from build123d import *

# Parameters (mm, degrees)
SKETCH1_R           = 11.1125
BOSS_EXTRUDE1_DEPTH = 38.1
SKETCH2_R           = 6.35
CUT_EXTRUDE1_DEPTH  = 25.4
SKETCH3_W           = 3.175
SKETCH3_H           = 1.5875
CUT_EXTRUDE2_DEPTH  = 25.4
CHAMFER2_SIZE       = 0.635
CHAMFER3_SIZE       = 1.27


with BuildPart() as part:
    # Sketch1 → Boss-Extrude1 (new body)
    with BuildSketch(Plane(origin=(0, 0, 0), x_dir=(0, 0, -1), z_dir=(1, 0, 0))):
        with Locations(Location((0, 0, 0), (0, 0, 180))):
            Circle(SKETCH1_R)
    extrude(amount=BOSS_EXTRUDE1_DEPTH)

    # Sketch2 → Cut-Extrude1 (cut)
    with BuildSketch(Plane(origin=(38.1, 0, 0), x_dir=(0, 0, -1), z_dir=(1, 0, 0))):
        Circle(SKETCH2_R)
    extrude(amount=-CUT_EXTRUDE1_DEPTH, mode=Mode.SUBTRACT)

    # Sketch3 → Cut-Extrude2 (cut)
    with BuildSketch(Plane(origin=(38.1, 0, 0), x_dir=(0, 0, -1), z_dir=(1, 0, 0))):
        with Locations((0, 6.35)):
            Rectangle(SKETCH3_W, SKETCH3_H)
    extrude(amount=-CUT_EXTRUDE2_DEPTH, mode=Mode.SUBTRACT)

    # Chamfer2
    chamfer2_edges = [part.edges().sort_by_distance(p)[0] for p in [
        (38.1, -6.35, 0),
    ]]
    chamfer(chamfer2_edges, length=CHAMFER2_SIZE)

    # Chamfer3
    chamfer3_edges = [part.edges().sort_by_distance(p)[0] for p in [
        (38.1, 0, -11.1125),
    ]]
    chamfer(chamfer3_edges, length=CHAMFER3_SIZE)


solid = part.part
Build history of the part. All positions in model axes, mm. A direction names the side the tool comes from. Give positions to 0.01 mm unless a question says otherwise; leave off trailing zeros. Put each result on its own line as item: value.
Item 1: Drop flat-ended pins along their axis: pin 1 Ø0.5 at (x, y) = (20.5, 6.5) entering from +Z; pin 2 Ø1.1 at (x, y) = (20.5, 6.5) entering from -Z; pin 3 Ø10 at (x, y) = (9.5, 6.5) entering from +Z. Give the stop position or say it passes through.
Results are:
pin 1: z = 9.19
pin 2: z = -9.39
pin 3: z = 11.01
Item 2: Which spindle directions (+Z, -Z, +X, -X, +Y, -Y) get a long thin tool onto all of the face, cutting with end or side? Do faces 1 (the face through (0, 0, 0)), 2 (the face through (12.7, 0, 0)). Say none if no direction does.
Results are:
face 1: +Z, -Z, -X, +Y, -Y
face 2: +X
Item 3: Pull direction Y, two halves, no side cores. Call faces 3 (the face through (38.1, -7, 2)), 4 (the face through (25.6, 6.6, 1.588)), 5 (the face through (25.256, -6.345, 0.257)), 6 (the face through (18.2, -7.5, -8.2)): +Y half, -Y half, draft (parallel to the pull), parting line (faces both ways), or undercut.
Results are:
face 3: draft
face 4: undercut
face 5: undercut
face 6: parting line
Item 4: Wall check: probe 1 along Y at (x, z) = (31, 0); probe 2 along Y at (x, z) = (17.5, 4.5); probe 3 along Z at (x, y) = (36.5, 2.25). Give the ranges that are in metal, low to high.
Results are:
probe 1: -11.11 to -6.35, 7.14 to 11.11
probe 2: -10.16 to -4.48, 4.48 to 10.16
probe 3: -10.88 to -5.94, 5.94 to 10.88
